Check sheet for the modelled part. Datum: model origin and axes. Units: mm. A direction names the side the tool comes from. Coordinates: 2 decimals unless noted, no trailing zeros. Write each loop counter-clockwise with the first axis right and the second up, starting at its lowest first coordinate (ties: lowest second). Pieces come first, ordered by that corner, then holes. Notation, with made-up numbers: (53.5, -0.5) - (84.5, -0.5) arc R26 ccw to (84.5, 23.5) - close; hole circle Ø3 at (67, 57.5). An arc over 180 degrees is marked (long way). Write each question's results on one line, items separated by ' | '.
from build123d import *

# Parameters (mm, degrees)
SKETCH1_R           = 2
BOSS_EXTRUDE1_DEPTH = 4
SKETCH2_W           = 4
SKETCH2_H           = 15
CUT_EXTRUDE1_DEPTH  = 3
SKETCH3_W           = 2.5
SKETCH3_H           = 20
CUT_EXTRUDE2_DEPTH  = 1
CUT_EXTRUDE3_REACH  = 10
SKETCH5_R           = 9


with BuildPart() as part:
    # Sketch1 → Boss-Extrude1 (new body, symmetric)
    with BuildSketch(Plane.XY):
        Polygon((-20, -17.5), (35, -17.5), (35, 17.5), (-35, 17.5), (-35, -7.5), (-20, -7.5), align=None)
        with BuildLine():
            ThreePointArc((31.5, -9), (28.939339828, -10.060660172), (30, -7.5))
            ThreePointArc((30, -7.5), (31.060660172, -7.939339828), (31.5, -9))
        make_face(mode=Mode.SUBTRACT)
        with Locations((-30, 12)):
            Circle(SKETCH1_R, mode=Mode.SUBTRACT)
        with BuildLine():
            ThreePointArc((31.5, 9), (31.060660172, 7.939339828), (30, 7.5))
            ThreePointArc((30, 7.5), (28.939339828, 10.060660172), (31.5, 9))
        make_face(mode=Mode.SUBTRACT)
    extrude(amount=BOSS_EXTRUDE1_DEPTH, both=True)

    # Sketch2 → Cut-Extrude1 (cut)
    with BuildSketch(Plane.XY.offset(4)):
        with Locations((-33, 0)):
            Rectangle(SKETCH2_W, SKETCH2_H)
    extrude(amount=-CUT_EXTRUDE1_DEPTH, mode=Mode.SUBTRACT)

    # Sketch3 → Cut-Extrude2 (cut)
    with BuildSketch(Plane(origin=(0, 0, -4), x_dir=(-1, 0, 0), z_dir=(0, 0, -1))):
        with Locations((-33.75, 0)):
            Rectangle(SKETCH3_W, SKETCH3_H)
    extrude(amount=-CUT_EXTRUDE2_DEPTH, mode=Mode.SUBTRACT)

    # Sketch5 → Cut-Extrude3 (cut, up to next)
    with BuildSketch(Plane.XY.offset(4), mode=Mode.PRIVATE) as cut_extrude3_sk1:
        with Locations((40, 0)):
            Circle(SKETCH5_R)
    cut_extrude3_tool1 = extrude(cut_extrude3_sk1.sketch, amount=-CUT_EXTRUDE3_REACH, mode=Mode.PRIVATE) & part.part
    add(cut_extrude3_tool1.solids().sort_by_distance((40, 0, 4))[0], mode=Mode.SUBTRACT)


solid = part.part
1. Go/stop test with flat-tipped pins: pin 1 (1.5 mm diameter, centred on y = -2, z = 2.5, fed in from -X); pin 2 (3.5 mm diameter, centred on x = -30, y = 12, fed in from -Z); pin 3 (4 mm diameter, centred on x = -24, z = -1, fed in from -Y); pin 4 (3 mm diameter, centred on x = 33.5, y = 7.5, fed in from -Z). Record where each tip stops, or that it passes through.
Values follow:
pin 1: stops at x = -31 | pin 2: passes through | pin 3: stops at y = -7.5 | pin 4: stops at z = -4
2. Sectioned sample at A-A (y = 9). Record the cut outline in (x, z), then the cut area to 4 significant figures.
Values follow:
outline: (-35, -4) - (28.5, -4) - (28.5, 4) - (-35, 4) - close; (31.5, -4) - (32.5, -4) - (32.5, -3) - (35, -3) - (35, 4) - (31.5, 4) - close | area: 533.5 mm^2
3. Material ranges on L1, parallel to Y at x = 30, z = -2.2; L2, parallel to Y at x = 29.5, z = -3.25; L3, parallel to X at y = -9, z = -0.9, recorded low to high. Write a range as [from, to].
Values follow:
L1: y = [-17.5, -10.5], [-7.5, 7.5], [10.5, 17.5] | L2: y = [-17.5, -10.41], [-7.59, 7.59], [10.41, 17.5] | L3: x = [-20, 28.5], [31.5, 35]
4. Access from +Z, -Z, +X, -X, +Y, -Y to the whole of each face (thin tool, end or side, straight path). Record for faces 1 (the flat face through (33, 8, -3)), 2 (the flat face through (-20, -12, 0)), 3 (the cylindrical face through (31.43, 8.55, -0.06)), 4 (the flat face through (0, 17.5, 0)), 5 (the flat face through (-33, 7.5, 3)).
Values follow:
face 1: -Z, +X | face 2: +Z, -Z, -X, -Y | face 3: +Z, -Z | face 4: +Z, -Z, +X, -X, +Y | face 5: +Z, -X, -Y
5. Sectioned sample at D-D (y = 3.5). Record the cut outline in (x, z), then the cut area to 3 significant figures.
Values follow:
outline: (-35, -4) - (31.71, -4) - (31.71, 4) - (-31, 4) - (-31, 1) - (-35, 1) - close | area: 522 mm^2
6. Draft check along Y on faces 6 (the flat face through (0, 0, -4)), 7 (the flat face through (33, -8, -3)), 8 (the flat face through (-28, -7.5, 0)). Enter one of: pulls with the +Y half, pulls with the -Y half, needs draft (parallel to the pull), parting line crosses it, or undercut.
Values follow:
face 6: needs draft | face 7: undercut | face 8: pulls with the -Y half
7. Sectioned sample at C-C (x = -24). Record the cut outline in (y, z).
Values follow:
outline: (-7.5, -4) - (17.5, -4) - (17.5, 4) - (-7.5, 4) - close
8. Sectioned sample at B-B (z = 2.5). Record the cut outline in (x, y), then the cut area to 3 significant figures.
Values follow:
outline: (-35, 7.5) - (-31, 7.5) - (-31, -7.5) - (-20, -7.5) - (-20, -17.5) - (35, -17.5) - (35, -7.48) arc R9 cw to (35, 7.48) - (35, 17.5) - (-35, 17.5) - close; hole circle Ø4 at (-30, 12); hole circle Ø3 at (30, -9); hole circle Ø3 at (30, 9) | area: 2,170 mm^2
